from build123d import *

# Parameters (mm, degrees)
BOSS_EXTRUDE1_DEPTH     = 2.1
CUT_EXTRUDE1_DEPTH      = 1.3
SKETCH3_R               = 1.1
CUT_EXTRUDE2_DEPTH      = 10.780593029
CUT_EXTRUDE3_DEPTH      = 10.573922916
CUT_EXTRUDE3_DEPTH_BACK = 10.573922916
SKETCH4_W               = 7.5
SKETCH4_H               = 1.9
SKETCH5_R               = 1
CUT_EXTRUDE4_DEPTH      = 10.810708435


with BuildPart() as part:
    # Sketch1 → Boss-Extrude1 (new, symmetric)
    with BuildSketch(Plane.XY):
        with BuildLine():
            Line((6.5, -2.5), (-6.5, -2.5))
            ThreePointArc((-6.5, -2.5), (-9, 0), (-6.5, 2.5))
            Line((-6.5, 2.5), (6.5, 2.5))
            ThreePointArc((6.5, 2.5), (9, 0), (6.5, -2.5))
        make_face()
    extrude(amount=BOSS_EXTRUDE1_DEPTH, both=True)

    # Sketch2 → Cut-Extrude1 (cut)
    with BuildSketch(Plane.XY.offset(2.1)):
        with BuildLine():
            Line((6.5, 2.5), (1.5, 2.5))
            ThreePointArc((1.5, 2.5), (4, 0), (1.5, -2.5))
            Line((1.5, -2.5), (6.5, -2.5))
            ThreePointArc((6.5, -2.5), (9, 0), (6.5, 2.5))
        make_face()
    extrude(amount=-CUT_EXTRUDE1_DEPTH, mode=Mode.SUBTRACT)

    # Sketch3 → Cut-Extrude2 (cut, through all)
    with BuildSketch(Plane.XY.offset(0.8)):
        with Locations((6.5, 0)):
            Circle(SKETCH3_R)
    extrude(amount=-CUT_EXTRUDE2_DEPTH, mode=Mode.SUBTRACT)

    # Sketch4 → Cut-Extrude3 (cut, two sides: drawn at the far end of the back side and taken through both)
    with BuildSketch(Plane(origin=(0, 0, 0), x_dir=(1, 0, 0), z_dir=(0, 1, 0)).offset(-CUT_EXTRUDE3_DEPTH_BACK)):
        with Locations((-5.25, -0.05)):
            Rectangle(SKETCH4_W, SKETCH4_H)
    extrude(amount=CUT_EXTRUDE3_DEPTH + CUT_EXTRUDE3_DEPTH_BACK, mode=Mode.SUBTRACT)

    # Sketch5 → Cut-Extrude4 (cut, through all)
    with BuildSketch(Plane.XY.offset(-0.9)):
        with Locations((-6.5, 0)):
            Circle(SKETCH5_R)
    extrude(amount=-CUT_EXTRUDE4_DEPTH, mode=Mode.SUBTRACT)


solid = part.part
Source: CAD feature listing. Evaluate the final solid. Frame: model axes, mm. A direction names the side the tool comes from. Give positions to 0.01 mm unless a question says otherwise; leave off trailing zeros. Order: outer loops, then holes, each group sorted by start corner. A loop starts at its lowest first (then second) coordinate and runs counter-clockwise, first axis right, second up. Notation, with made-up numbers: (80, 59.25) -> (99, 59.25) arc R21 ccw to (99, 83.25) -> close; hole circle Ø2 at (55, 25). An arc over 180 degrees is marked (long way). Use a Markdown table: item, result.
1) Section query A-A, the plane y = 0. Return the cut outline in (x, z), then the cut area to 3 significant figures.
Answer list:
| item | result |
|---|---|
| outline | (-9, -2.1) -> (-7.5, -2.1) -> (-7.5, -0.9) -> (-9, -0.9) -> close; (-9, 1) -> (-1.5, 1) -> (-1.5, -0.9) -> (-5.5, -0.9) -> (-5.5, -2.1) -> (5.4, -2.1) -> (5.4, 0.8) -> (4, 0.8) -> (4, 2.1) -> (-9, 2.1) -> close; (7.6, -2.1) -> (9, -2.1) -> (9, 0.8) -> (7.6, 0.8) -> close |
| area | 46.1 mm² |
2) Section query D-D, the plane x = -6. Return the cut outline in (y, z), then the cut area to 3 significant figures.
Answer list:
| item | result |
|---|---|
| outline | (-2.5, -2.1) -> (-0.87, -2.1) -> (-0.87, -0.9) -> (-2.5, -0.9) -> close; (-2.5, 1) -> (2.5, 1) -> (2.5, 2.1) -> (-2.5, 2.1) -> close; (0.87, -2.1) -> (2.5, -2.1) -> (2.5, -0.9) -> (0.87, -0.9) -> close |
| area | 9.42 mm² |
3) Ray query, line 1 along Z through (x, y) = (-5, -0.65); line 2 along Y through (x, z) = (-6.5, -1.75); line 3 along Y through (x, z) = (6.5, 0.05). Return the intervals inside material, ascending. Write a range as [from, to].
Answer list:
| item | result |
|---|---|
| line 1 | [-2.1, -0.9], [1, 2.1] |
| line 2 | [-2.5, -1], [1, 2.5] |
| line 3 | [-2.5, -1.1], [1.1, 2.5] |
4) Mould query, pull axis Z, two halves, no side actions, for faces 4 (the flat face through (5, 0, 0.8)), 5 (the flat face through (-1.5, 0, 0)), 6 (the cylindrical face through (9, 0, -1)). Classes: +Z half, -Z half, draft (parallel to the pull), parting line (faces both ways), or undercut.
Answer list:
| item | result |
|---|---|
| face 4 | +Z half |
| face 5 | undercut |
| face 6 | draft |
5) Reachability of faces 1 (the cylindrical face through (-7.3, -0.6, -1.5)), 2 (the flat face through (-5, 0, 1)), 3 (the cylindrical face through (4, 0, 1)) from +Z, -Z, +X, -X, +Y, -Y: full face, straight path, thin tool, end or side. Return the list, or none.
Answer list:
| item | result |
|---|---|
| face 1 | -Z |
| face 2 | -X, +Y, -Y |
| face 3 | +Z, +X |
6) Contact query for a flat-ended pin moving along its axis: P1, Ø2, axis at y = -1, z = 0, coming from the -X side. Output: stop coordinate, or through.
Answer list:
| item | result |
|---|---|
| P1 | x = -8.94 |
7) Section query B-B, the plane x = -2.5. Return the cut outline in (y, z), then the cut area to 3 significant figures.
Answer list:
| item | result |
|---|---|
| outline | (-2.5, -2.1) -> (2.5, -2.1) -> (2.5, -0.9) -> (-2.5, -0.9) -> close; (-2.5, 1) -> (2.5, 1) -> (2.5, 2.1) -> (-2.5, 2.1) -> close |
| area | 11.5 mm² |
8) Section query C-C, the plane z = -1.25. Return the cut outline in (x, y), then the cut area to 3 significant figures.
Answer list:
| item | result |
|---|---|
| outline | (-6.5, -2.5) -> (6.5, -2.5) arc R2.5 ccw to (6.5, 2.5) -> (-6.5, 2.5) arc R2.5 ccw to start; hole circle Ø2 at (-6.5, 0); hole circle Ø2.2 at (6.5, 0) |
| area | 77.7 mm² |
